Build history of the part. All positions in model axes, mm. A direction names the side the tool comes from. Give positions to 0.01 mm unless a question says otherwise; leave off trailing zeros. Order: outer loops, then holes, each group sorted by start corner. A loop starts at its lowest first (then second) coordinate and runs counter-clockwise, first axis right, second up. Notation, with made-up numbers: (-11.5, 1.5) -> (37.5, 1.5) arc R18 ccw to (37.5, 18.5) -> close; hole circle Ø6 at (27.25, 72). An arc over 180 degrees is marked (long way). One line per question, with ' | ' between items. Start each with the question number.
(1) Cut at B-B (y = 4.5). Give the cut face in (x, z), then the cut area to 3 significant figures.
(2) Pin check, flat tips, straight feed: pin 1 Ø11 at (x, z) = (-17, 4) entering from -Y; pin 2 Ø9 at (x, z) = (15, 1.8) entering from -Y; pin 3 Ø2 at (y, z) = (5, -5.5) entering from -X; pin 4 Ø2.5 at (x, z) = (-15, 1.8) entering from -Y. Stop position of each tip, or through.
(3) Pull direction X, two halves, no side cores. Call faces 4 (the face through (-17.196, 5.535, 1.316)), 5 (the face through (16.5, 4, -18)), 6 (the face through (0, 0, -3)): +X half, -X half, draft (parallel to the pull), parting line (faces both ways), or undercut.
(4) Cut at A-A (x = 15). Give the cut face in (y, z), then the cut area to 4 significant figures.
(5) Cut at D-D (y = 1.25). Give the cut face in (x, z).
(6) Cut at C-C (z = 5.5). Give the cut face in (x, y), then the cut area to 3 significant figures.
(7) Which spindle directions (+Z, -Z, +X, -X, +Y, -Y) get a long thin tool onto all of the face, cutting with end or side? Do faces 1 (the face through (6.993, -1.014, -6.778)), 2 (the face through (-7.148, -1.014, -6.933)), 3 (the face through (-17.2, 3, 0.8)). Say none if no direction does.
(8) Drill centre lines: L1, parallel to X at y = 4.5, z = -13.5; L2, parallel to Y at x = 15, z = -13; L3, parallel to Y at x = -14, z = -2.5. Where is each one in solid material? Low to high. Write a range as from..to.
from build123d import *

# Parameters (mm, degrees)
BOSS_EXTRUDE1_DEPTH                     = 8
SKETCH2_W                               = 20
SKETCH2_H                               = 20
BOSS_EXTRUDE2_DEPTH                     = 2
FILLET1_R                               = 10
SKETCH3_R                               = 7.29
CUT_EXTRUDE1_DEPTH                      = 37.020349658
CUT_EXTRUDE1_DRAFT                      = 4
CBORE_FOR_M5_HEX_HEAD_BOLT1_D           = 4.5
CBORE_FOR_M5_HEX_HEAD_BOLT1_CBORE_D     = 10
CBORE_FOR_M5_HEX_HEAD_BOLT1_CBORE_DEPTH = 3


with BuildPart() as part:
    # Sketch1 → Boss-Extrude1 (new body)
    with BuildSketch(Plane(origin=(0, 0, 0), x_dir=(1, 0, 0), z_dir=(0, 1, 0))):
        Polygon((-25, 3.926253144), (-25, -11.073746856), (25, -11.073746856), (25, 3.926253144), (16.5, 12.426253144), (16.5, 23.926253144), (-16.5, 23.926253144), (-16.5, 12.426253144), align=None)
    extrude(amount=BOSS_EXTRUDE1_DEPTH)

    # Sketch2 → Boss-Extrude2 (add)
    with BuildSketch(Plane.XZ):
        with Locations((0, -13.926253144)):
            Rectangle(SKETCH2_W, SKETCH2_H)
    extrude(amount=BOSS_EXTRUDE2_DEPTH)

    # Fillet1
    fillet1_edges = [part.edges().sort_by_distance(p)[0] for p in [
        (-10, -1, -3.926253144),
        (10, -1, -3.926253144),
    ]]
    fillet(fillet1_edges, radius=FILLET1_R - 0.0001)  # a hair under: the kernel refuses the full size


with BuildPart() as cut_extrude1_tool:
    # Sketch3 → Cut-Extrude1 (with draft: the straight prism first)
    with BuildSketch(Plane.XZ.offset(2)):
        with Locations((0, -22.926253144)):
            Circle(SKETCH3_R)
    extrude(amount=-CUT_EXTRUDE1_DEPTH)
    # Cut-Extrude1: the draft: its side faces are tilted about the plane it starts from
    cut_extrude1_sides = [cut_extrude1_tool.faces().sort_by_distance(p)[0] for p in [
        (-7.29, 16.510174829, -22.926253144),
    ]]
    draft(cut_extrude1_sides, Plane.XZ.offset(2), CUT_EXTRUDE1_DRAFT)


with BuildPart() as part_1:
    add(part.part)

    # Cut-Extrude1: cut by cut_extrude1_tool
    add(cut_extrude1_tool.part, mode=Mode.SUBTRACT)

    # CBORE for M5 Hex Head Bolt1 (through all)
    with Locations(Plane(origin=(-15, 0, 1.804006093), x_dir=(0, 0, -1), z_dir=(0, -1, 0))):
        with Locations((0, 0), (0, 30)):
            CounterBoreHole(CBORE_FOR_M5_HEX_HEAD_BOLT1_D / 2, CBORE_FOR_M5_HEX_HEAD_BOLT1_CBORE_D / 2, CBORE_FOR_M5_HEX_HEAD_BOLT1_CBORE_DEPTH)


solid = part_1.part
Result set:
1) outline: (-25, -3.93) -> (-16.5, -12.43) -> (-16.5, -23.93) -> (-7.68, -23.93) arc R7.74 cw (long way) to (7.68, -23.93) -> (16.5, -23.93) -> (16.5, -12.43) -> (25, -3.93) -> (25, 11.07) -> (-25, 11.07) -> close; hole circle Ø4.5 at (-15, 1.8); hole circle Ø4.5 at (15, 1.8) | area: 1,340 mm2
2) pin 1: stops at y = 0 | pin 2: stops at y = 3 | pin 3: stops at x = -24.43 | pin 4: passes through
3) face 4: undercut | face 5: +X half | face 6: draft
4) outline: (0, -23.93) -> (8, -23.93) -> (8, -0.45) -> (3, -0.45) -> (3, -3.2) -> (0, -3.2) -> close; (0, 6.8) -> (3, 6.8) -> (3, 4.05) -> (8, 4.05) -> (8, 11.07) -> (0, 11.07) -> close | area: 227.5 mm2
5) outline: (-25, -3.93) -> (-16.5, -12.43) -> (-16.5, -23.93) -> (-7.45, -23.93) arc R7.52 cw (long way) to (7.45, -23.93) -> (16.5, -23.93) -> (16.5, -12.43) -> (25, -3.93) -> (25, 11.07) -> (-25, 11.07) -> close; hole circle Ø10 at (-15, 1.8); hole circle Ø10 at (15, 1.8)
6) outline: (-25, 0) -> (-18.37, 0) -> (-18.37, 3) -> (-11.63, 3) -> (-11.63, 0) -> (11.63, 0) -> (11.63, 3) -> (18.37, 3) -> (18.37, 0) -> (25, 0) -> (25, 8) -> (-25, 8) -> close | area: 360 mm2
7) face 1: +Z, +X, -Y | face 2: +Z, -X, -Y | face 3: -Y
8) L1: x = -16.5..16.5 | L2: y = 0..8 | L3: y = 3..8
